Here's how the part is built. I have some questions about the finished solid (model axes, mm). A direction names the side the tool comes from. Give positions to 0.01 mm unless a question says otherwise; leave off trailing zeros. Write each loop counter-clockwise with the first axis right and the second up, starting at its lowest first coordinate (ties: lowest second). Pieces come first, ordered by that corner, then holes. Notation, with made-up numbers: (9, 87) -> (45, 87) arc R17 ccw to (45, 119) -> close; hole circle Ø10 at (22, 33). An arc over 180 degrees is marked (long way). Use one line per item in the form item = value.
```python
from build123d import *

# Parameters (mm, degrees)
SKETCH1_W                                    = 50
SKETCH1_H                                    = 50
BOSS_EXTRUDE1_DEPTH                          = 10
SHELL1_T                                     = -2.5
FILLET1_R                                    = 5
SKETCH2_W                                    = 6
SKETCH2_H                                    = 6
BOSS_EXTRUDE2_DEPTH                          = 9.5
CSK_SLOT_FOR_M1_6_COUNTERSUNK_FLAT_H_2_COUNT = 2
CSK_SLOT_FOR_M1_6_COUNTERSUNK_FLAT_H_2_PITCH = 40
CSK_SLOT_FOR_M1_6_COUNTERSUNK_FLAT_H_3_COUNT = 2
CSK_SLOT_FOR_M1_6_COUNTERSUNK_FLAT_H_3_PITCH = 56.568542495
CSK_SLOT_FOR_M1_6_COUNTERSUNK_FLAT_H_4_COUNT = 2
CSK_SLOT_FOR_M1_6_COUNTERSUNK_FLAT_H_4_PITCH = 40
SKETCH7_W                                    = 12
SKETCH7_H                                    = 23
BOSS_EXTRUDE3_DEPTH                          = 6
SKETCH8_W                                    = 2
SKETCH8_H                                    = 3
CUT_EXTRUDE1_DEPTH                           = 43.72294479
FILLET2_R                                    = 1
SKETCH9_W                                    = 4.34
SKETCH9_H                                    = 1.8
CUT_EXTRUDE2_DEPTH                           = 4.4
SKETCH10_W                                   = 3.1
SKETCH10_H                                   = 1.1
CUT_EXTRUDE3_DEPTH                           = 3.55
CUT_EXTRUDE4_REACH                           = 40.194
SKETCH13_W                                   = 3.1
SKETCH13_H                                   = 2
FILLET3_R                                    = 2


with BuildPart() as part:
    # Sketch1 → Boss-Extrude1 (new body)
    with BuildSketch(Plane(origin=(0, 0, 0), x_dir=(1, 0, 0), z_dir=(0, 1, 0))):
        Rectangle(SKETCH1_W, SKETCH1_H)
    extrude(amount=BOSS_EXTRUDE1_DEPTH)

    # Shell1
    shell1_openings = [part.faces().sort_by_distance(p)[0] for p in [
        (0, 10, 0),
    ]]
    offset(amount=SHELL1_T, openings=shell1_openings, kind=Kind.INTERSECTION)

    # Fillet1
    fillet1_edges = [part.edges().sort_by_distance(p)[0] for p in [
        (0, 0, 25),
        (-25, 0, 0),
        (0, 0, -25),
        (25, 0, 0),
        (25, 5, 25),
        (-25, 5, 25),
        (-25, 5, -25),
        (25, 5, -25),
    ]]
    fillet(fillet1_edges, radius=FILLET1_R)

    # Sketch2 → Boss-Extrude2 (add)
    with BuildSketch(Plane(origin=(0, 2.5, 0), x_dir=(1, 0, 0), z_dir=(0, 1, 0))):
        with Locations((19.5, 19.5)):
            Rectangle(SKETCH2_W, SKETCH2_H)
        with Locations((-19.5, 19.5)):
            Rectangle(SKETCH2_W, SKETCH2_H)
        with Locations((19.5, -19.5)):
            Rectangle(SKETCH2_W, SKETCH2_H)
        with Locations((-19.5, -19.5)):
            Rectangle(SKETCH2_W, SKETCH2_H)
    extrude(amount=BOSS_EXTRUDE2_DEPTH)

    # Sketch6 → CSK SLOT for M1.6 Countersunk Flat Head Screw1 (revolve, cut)
    with BuildSketch(Plane(origin=(20, 0, 20), x_dir=(0, 0, -1), z_dir=(1, 0, 0))):
        Polygon((0, 0), (0, 12), (0.9, 12), (0.9, 10.9), (1.8, 10), (1.8, 0), align=None)
    csk_slot_for_m1_6_countersunk_flat_head = revolve(axis=Axis((20, -6.35, 20), (0, 1, 0)), mode=Mode.SUBTRACT)

    # CSK SLOT for M1.6 Countersunk Flat H 2: CSK SLOT for M1.6 Countersunk Flat Head Screw1 ×2
    with Locations(*[(-i * CSK_SLOT_FOR_M1_6_COUNTERSUNK_FLAT_H_2_PITCH, 0, 0) for i in range(1, CSK_SLOT_FOR_M1_6_COUNTERSUNK_FLAT_H_2_COUNT)]):
        add(csk_slot_for_m1_6_countersunk_flat_head, mode=Mode.SUBTRACT)

    # CSK SLOT for M1.6 Countersunk Flat H 3: CSK SLOT for M1.6 Countersunk Flat Head Screw1 ×2
    with Locations(*[Vector(-0.7071067811865476, 0, -0.7071067811865475) * (i * CSK_SLOT_FOR_M1_6_COUNTERSUNK_FLAT_H_3_PITCH) for i in range(1, CSK_SLOT_FOR_M1_6_COUNTERSUNK_FLAT_H_3_COUNT)]):
        add(csk_slot_for_m1_6_countersunk_flat_head, mode=Mode.SUBTRACT)

    # CSK SLOT for M1.6 Countersunk Flat H 4: CSK SLOT for M1.6 Countersunk Flat Head Screw1 ×2
    with Locations(*[(0, 0, -i * CSK_SLOT_FOR_M1_6_COUNTERSUNK_FLAT_H_4_PITCH) for i in range(1, CSK_SLOT_FOR_M1_6_COUNTERSUNK_FLAT_H_4_COUNT)]):
        add(csk_slot_for_m1_6_countersunk_flat_head, mode=Mode.SUBTRACT)

    # Sketch7 → Boss-Extrude3 (add)
    with BuildSketch(Plane.XZ):
        with Locations((0, 4)):
            Rectangle(SKETCH7_W, SKETCH7_H)
    extrude(amount=BOSS_EXTRUDE3_DEPTH)

    # Sketch8 → Cut-Extrude1 (cut, through all)
    with BuildSketch(Plane(origin=(0, 0, -7.5), x_dir=(-1, 0, 0), z_dir=(0, 0, -1))):
        with Locations((5, -1.5)):
            Rectangle(SKETCH8_W, SKETCH8_H)
        with Locations((-5, -1.5)):
            Rectangle(SKETCH8_W, SKETCH8_H)
    extrude(amount=-CUT_EXTRUDE1_DEPTH, mode=Mode.SUBTRACT)

    # Fillet2
    fillet2_edges = [part.edges().sort_by_distance(p)[0] for p in [
        (-6, -4.5, -7.5),
        (6, -4.5, -7.5),
        (0, -6, -7.5),
    ]]
    fillet(fillet2_edges, radius=FILLET2_R)

    # Sketch9 → Cut-Extrude2 (cut)
    with BuildSketch(Plane(origin=(0, 0, -7.5), x_dir=(-1, 0, 0), z_dir=(0, 0, -1))):
        with Locations((0, -3)):
            Rectangle(SKETCH9_W, SKETCH9_H)
    extrude(amount=-CUT_EXTRUDE2_DEPTH, mode=Mode.SUBTRACT)

    # Sketch10 → Cut-Extrude3 (cut)
    with BuildSketch(Plane(origin=(0, 0, -3.1), x_dir=(-1, 0, 0), z_dir=(0, 0, -1))):
        with Locations((0, -3)):
            Rectangle(SKETCH10_W, SKETCH10_H)
    extrude(amount=-CUT_EXTRUDE3_DEPTH, mode=Mode.SUBTRACT)

    # Sketch13 → Cut-Extrude4 (cut, up to next)
    with BuildSketch(Plane.XZ.offset(2.45), mode=Mode.PRIVATE) as cut_extrude4_sk1:
        with Locations((0, -0.55)):
            Rectangle(SKETCH13_W, SKETCH13_H)
    cut_extrude4_tool1 = extrude(cut_extrude4_sk1.sketch, amount=-CUT_EXTRUDE4_REACH, mode=Mode.PRIVATE) & part.part
    add(cut_extrude4_tool1.solids().sort_by_distance((0, -2.45, -0.55))[0], mode=Mode.SUBTRACT)

    # Fillet3
    fillet3_edges = [part.edges().sort_by_distance(p)[0] for p in [
        (-22.5, 11, 22.5),
        (-22.5, 11, -22.5),
        (22.5, 11, -22.5),
        (22.5, 11, 22.5),
    ]]
    fillet(fillet3_edges, radius=FILLET3_R)


solid = part.part
```
Q1. If we mould it in two halves opening along X, with no side actions, what happens to faces 1 (the face through (0, -3, 15.5)), 2 (the face through (0, 6, 22.5)), 3 (the face through (-4, -2, 4))? For each: +X half, -X half, draft (parallel to the pull), parting line (faces both ways), or undercut.
Result set:
face_1 = draft
face_2 = undercut
face_3 = -X half
Q2. If I drill on line 1 along Z through (x, y) = (20, 11.65); line 2 along Z through (x, y) = (-20, 7.75), over which ranges is the centre line in solid material (lowest first)? Write a range as from..to.
Result set:
line_1 = -22.5..-20.9, -19.1..-16.5, 16.5..19.1, 20.9..22.5
line_2 = -25..-21.8, -18.2..-16.5, 16.5..18.2, 21.8..25
Q3. I want a section at A-A, the plane x = 0.5. Write out the boundary of the cut face in (y, z), and give its area (3 significant figures).
Result set:
outline = (-6, -6.5) arc R1 ccw to (-5, -7.5) -> (-3.9, -7.5) -> (-3.9, -3.1) -> (-3.55, -3.1) -> (-3.55, 0.45) -> (2.5, 0.45) -> (2.5, 22.5) -> (10, 22.5) -> (10, 25) -> (5, 25) arc R5 ccw to (0, 20) -> (0, 15.5) -> (-6, 15.5) -> close; (-2.45, -3.1) -> (-2.1, -3.1) -> (-2.1, -7.5) -> (0, -7.5) -> (0, -20) arc R5 ccw to (5, -25) -> (10, -25) -> (10, -22.5) -> (2.5, -22.5) -> (2.5, -1.55) -> (-2.45, -1.55) -> close
area = 268 mm2
Q4. Which directions (+Z, -Z, +X, -X, +Y, -Y) give clear straight access to the entire face, cutting with the end or side of a thin tool? Please do faces 4 (the face through (-21.93, 11.01, 21.9)), 5 (the face through (0, -3.55, -1)), 6 (the face through (0, 0, -1.55)), 7 (the face through (-1.55, -1, -1)), 8 (the face through (-21.785, 4.93, 20.234)).
Result set:
face_4 = +Z, -X, +Y
face_5 = -Z
face_6 = +Y
face_7 = none
face_8 = -Y
Q5. Will these pins go through, and if not, where does the flat tip stop? pin 1 Ø6 at (y, z) = (0, -4) entering from -X; pin 2 Ø1.1 at (x, z) = (20, -20) entering from -Y; pin 3 Ø5 at (x, z) = (-13.5, -12.5) entering from +Y; pin 4 Ø3 at (x, y) = (-1, -2.5) entering from +Z.
Result set:
pin_1 = -24.58
pin_2 = through
pin_3 = 2.5
pin_4 = 15.5
Q6. I want a section at D-D, the plane x = -10. Write out the boundary of the cut face in (y, z), and give its area (3 significant figures).
Result set:
outline = (0, -20) arc R5 ccw to (5, -25) -> (10, -25) -> (10, -22.5) -> (2.5, -22.5) -> (2.5, 22.5) -> (10, 22.5) -> (10, 25) -> (5, 25) arc R5 ccw to (0, 20) -> close
area = 152 mm2
Q7. I want a section at C-C, the plane z = 8.5. Write out the boundary of the cut face in (x, y).
Result set:
outline = (-25, 5) arc R5 ccw to (-20, 0) -> (-4, 0) -> (-4, -3) -> (-6, -3) -> (-6, -6) -> (6, -6) -> (6, -3) -> (4, -3) -> (4, 0) -> (20, 0) arc R5 ccw to (25, 5) -> (25, 10) -> (22.5, 10) -> (22.5, 2.5) -> (-22.5, 2.5) -> (-22.5, 10) -> (-25, 10) -> close
Q8. I want a section at B-B, the plane y = -1.5. Write out the boundary of the cut face in (x, z).
Result set:
outline = (-4, -7.5) -> (4, -7.5) -> (4, 15.5) -> (-4, 15.5) -> close; hole (-1.55, -1.55) -> (1.55, -1.55) -> (1.55, 0.45) -> (-1.55, 0.45) -> close
